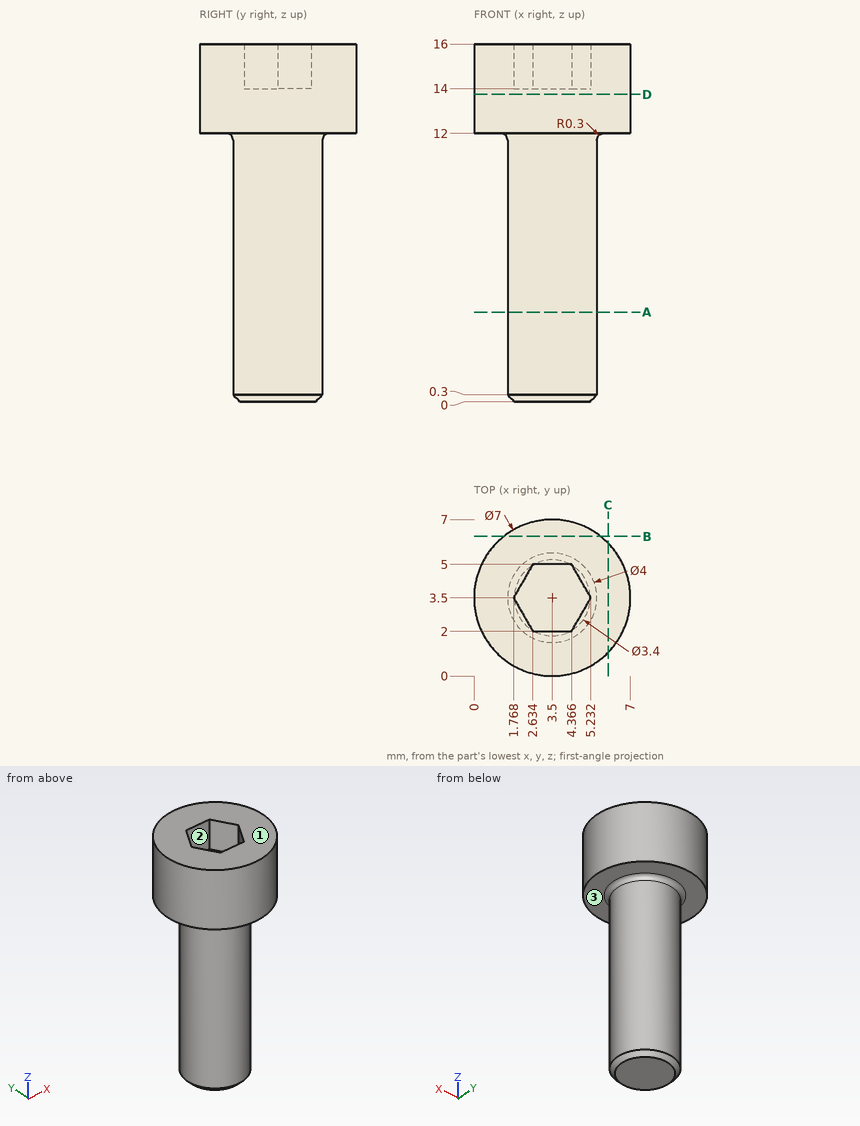
Geometry check sheet. Reference: drawing and pictorial views, mm from the part's lowest x, y, z. A direction names the side the tool comes from. Give positions to 0.01 mm unless a question says otherwise; leave off trailing zeros. Write each loop counter-clockwise with the first axis right and the second up, starting at its lowest first coordinate (ties: lowest second). Pieces come first, ordered by that corner, then holes.
Item 1: Cross-section at A-A (z = 4). Enter the section's corners in (x, y).
Item 2: Cross-section at C-C (x = 6). Enter the section's corners in (y, z).
Item 3: Access from +Z, -Z, +X, -X, +Y, -Y to the whole of each face (thin tool, end or side, straight path). Record for the marked faces 1, 2 and 3.
Item 4: Cross-section at B-B (y = 6.25). Enter the section's corners in (x, z) (3 decimals), and give its area (3 significant figures).
Item 5: Cross-section at D-D (z = 13.75). Enter the section's corners in (x, y).
Item 6: Scan lines: L1, parallel to Z at x = 5, y = 1; L2, parallel to Z at x = 3, y = 4; L3, parallel to X at y = 2.5, z = 4.25. Record each from-to range of solid material in increasing order.
Item 7: Gauge pin test, flat ends, axial feed: pin 1 (2 mm diameter, centred on x = 6.5, z = 13, fed in from +Y); pin 2 (1.5 mm diameter, centred on x = 3.5, y = 3.5, fed in from +Z); pin 3 (2 mm diameter, centred on y = 4.5, z = 11.5, fed in from +X). Record the tip position at first contact, or that the pin passes through.
Report:
1. outline: circle Ø4 at (3.5, 3.5)
2. outline: (1.05, 12) - (5.95, 12) - (5.95, 16) - (1.05, 16) - close
3. face 1: +Z, +X, -X, +Y, -Y
3. face 2: +Z
3. face 3: -Z
4. outline: (1.335, 12) - (5.665, 12) - (5.665, 16) - (1.335, 16) - close
4. area: 17.3 mm2
5. outline: circle Ø7 at (3.5, 3.5)
6. L1: z = 12 to 16
6. L2: z = 0 to 14
6. L3: x = 1.77 to 5.23
7. pin 1: stops at y = 6.37
7. pin 2: stops at z = 14
7. pin 3: stops at x = 7
